CAD build for the part. Positions are in the model's coordinates, mm. Round coordinates to 2 decimals unless told otherwise and drop trailing zeros. Loops run counter-clockwise (first coordinate to the right, second up) from the corner with the lowest first, then second, coordinate; pieces in that order, holes last.
from build123d import *

# Parameters (mm, degrees)
F1_DEPTH = 25.4
F2_R     = 6.35
F3_DEPTH = 25.4


with BuildPart() as f1:
    # F0 (on Top) → F1 (new body)
    with BuildSketch(Plane.XY):
        Polygon((76.2, 177.238014), (-76.2, 177.238014), (0, -117.883317), align=None)
    extrude(amount=F1_DEPTH)

    # F2 (on face) → F3 (cut)
    with BuildSketch(Plane.XY.offset(25.4)):
        with Locations((-57.170211, 164.495959)):
            Circle(F2_R)
        with Locations((57.170211, 164.495959)):
            Circle(F2_R)
    extrude(amount=-F3_DEPTH, mode=Mode.SUBTRACT)


solid = f1.part
Item 1: Cut at B-B (z = 12.75). List the corners of the cut face in (x, y).
Verdict:
outline: (-76.2, 177.24) - (0, -117.88) - (76.2, 177.24) - close; hole circle Ø12.7 at (-57.17, 164.5); hole circle Ø12.7 at (57.17, 164.5)
Item 2: Cut at D-D (y = 11). List the corners of the cut face in (x, z).
Verdict:
outline: (-33.28, 0) - (33.28, 0) - (33.28, 25.4) - (-33.28, 25.4) - close
Item 3: Wall check: L1, parallel to X at y = -26.5, z = 23.25; L2, parallel to X at y = -49, z = 18. Give the ranges that are in metal, low to high.
Verdict:
L1: x = -23.6 to 23.6
L2: x = -17.79 to 17.79
Item 4: Mould opens along X. For faces 1 (the flat face through (37.567, 27.611, 12.522)), 2 (the flat face through (-1, 65, 0)), 3 (the flat face through (-38.633, 31.743, 12.522)), 4 (the cylindrical face through (52.5, 168.8, 12.9)) say: released by +X, released by -X, zero draft, split by the parting line, or undercut.
Verdict:
face 1: released by +X
face 2: zero draft
face 3: released by -X
face 4: undercut
Item 5: Flat gauge pins, fed straight in: P1, Ø12, axis at y = -77.5, z = 13.5, coming from the -X side; P2, Ø2, axis at y = -18, z = 20, coming from the +X side. Where does each tip first touch, or does it go through?
Verdict:
P1: stops at x = -11.98
P2: stops at x = 26.05
Item 6: Cut at C-C (x = 59). List the corners of the cut face in (y, z), plus the area to 3 significant figures.
Verdict:
outline: (110.62, 0) - (158.42, 0) - (158.42, 25.4) - (110.62, 25.4) - close; (170.58, 0) - (177.24, 0) - (177.24, 25.4) - (170.58, 25.4) - close
area: 1,380 mm2
Item 7: Cut at A-A (x = -58.5). List the corners of the cut face in (y, z), plus the area to 3 significant figures.
Verdict:
outline: (108.69, 0) - (158.29, 0) - (158.29, 25.4) - (108.69, 25.4) - close; (170.71, 0) - (177.24, 0) - (177.24, 25.4) - (170.71, 25.4) - close
area: 1,430 mm2
